Drawing for the job (mm, zero at the part's lowest x, y, z). Coordinates: 2 decimals unless noted, no trailing zeros. Write each loop counter-clockwise with the first axis right and the second up, starting at its lowest first coordinate (ties: lowest second). Pieces come first, ordered by that corner, then holes. Notation, with made-up numbers: (83, 16) -> (115, 16) arc R28 ccw to (115, 35) -> close; hole circle Ø4 at (-4, -2). An arc over 180 degrees is marked (long way). Write each question's results on one line, items separated by ' | '. Start each with the question number.
Q1. Saw through at C-C on y = 88. Give the cut face in (x, z).
Q2. Drill centre lines: line 1 (Y direction, x = 12, z = 2.7); line 2 (Y direction, x = 134.5, z = 1.7); line 3 (X direction, y = 90.5, z = 2.5). Where is each one in solid material? Low to high.
Q3. Saw through at A-A on x = 12. Give the cut face in (y, z).
Q4. Saw through at B-B on z = 2.5. Give the cut face in (x, y).
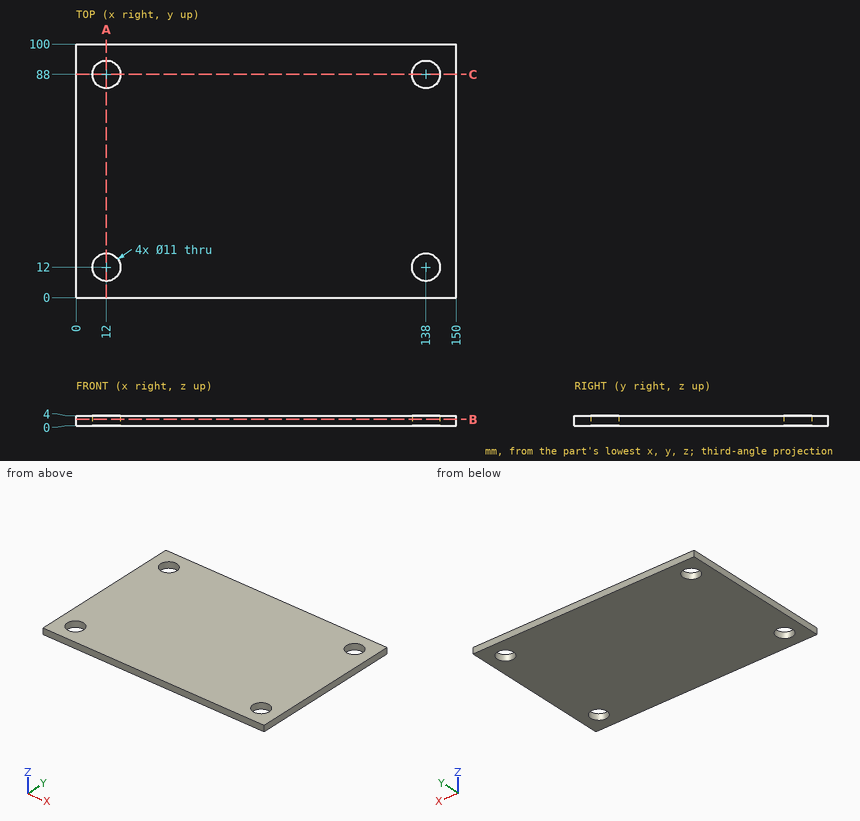
Returned:
1) outline: (0, 0) -> (6.5, 0) -> (6.5, 4) -> (0, 4) -> close; (17.5, 0) -> (132.5, 0) -> (132.5, 4) -> (17.5, 4) -> close; (143.5, 0) -> (150, 0) -> (150, 4) -> (143.5, 4) -> close
2) line 1: y = 0 to 6.5, 17.5 to 82.5, 93.5 to 100 | line 2: y = 0 to 7.76, 16.24 to 83.76, 92.24 to 100 | line 3: x = 0 to 7.1, 16.9 to 133.1, 142.9 to 150
3) outline: (0, 0) -> (6.5, 0) -> (6.5, 4) -> (0, 4) -> close; (17.5, 0) -> (82.5, 0) -> (82.5, 4) -> (17.5, 4) -> close; (93.5, 0) -> (100, 0) -> (100, 4) -> (93.5, 4) -> close
4) outline: (0, 0) -> (150, 0) -> (150, 100) -> (0, 100) -> close; hole circle Ø11 at (12, 12); hole circle Ø11 at (12, 88); hole circle Ø11 at (138, 12); hole circle Ø11 at (138, 88)
